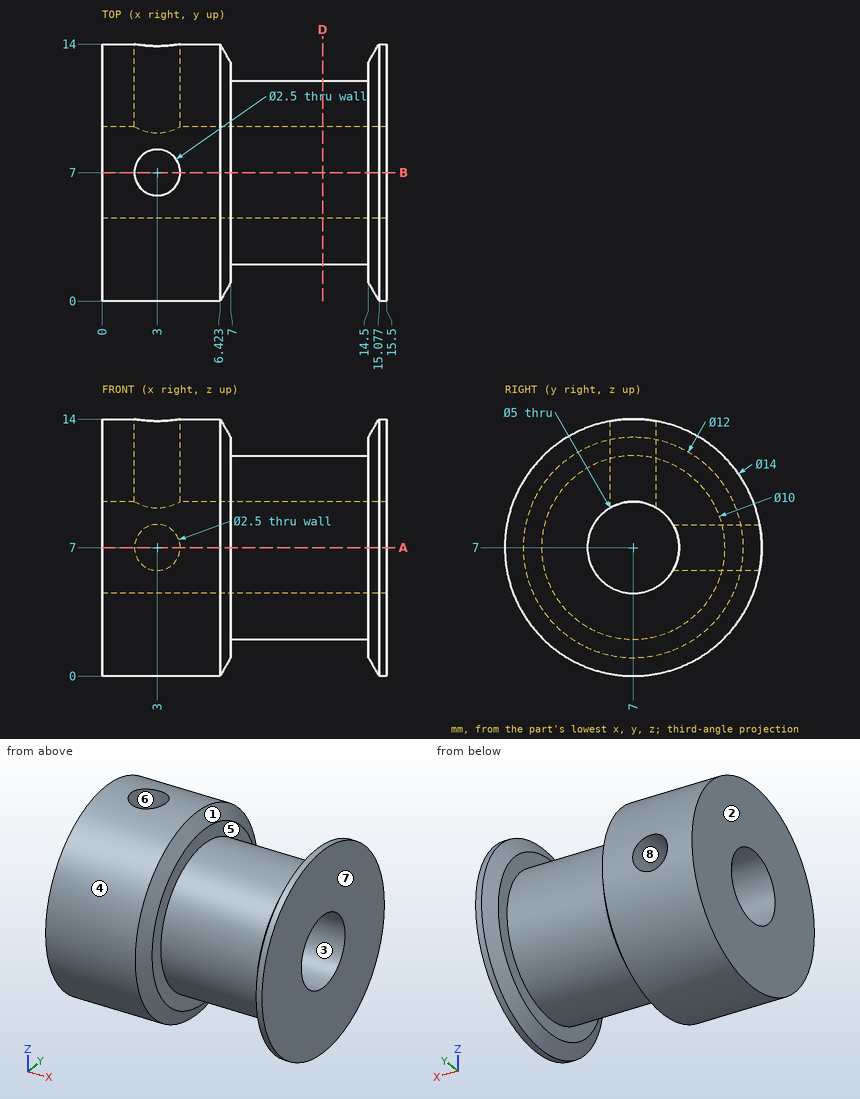
Verification items for this drawing (mm, ordinates from the low corner). A direction names the side the tool comes from. Give positions to 0.01 mm unless a question says otherwise; leave off trailing zeros. Loops run counter-clockwise (first coordinate to the right, second up) from the corner with the lowest first, then second, coordinate; pieces in that order, holes last. Notation, with made-up numbers: M 88.25,53 L 119.25,53 A16 cw 119.25,68 Z; hole C -25,73 d9. An arc over 180 degrees is marked long. Write item = value, one per line. Start each with the question number.
1. Draft check along Z on the marked faces 1, 2 and 3. Enter one of: +Z half, -Z half, draft (parallel to the pull), parting line (faces both ways), or undercut.
2. Section check A-A, the plane z = 7. Enter the section's corners in (x, y).
3. Go/stop test with flat-tipped pins: P1, Ø3, axis at x = 9.5, y = 8.5, coming from the +Z side; P2, Ø1.5, axis at x = 2.5, z = 12, coming from the -Y side. Record where each tip stops, or that it passes through.
4. Tool access check on the marked faces 4, 5, 6, 7 and 8. Record the directions out of +Z, -Z, +X, -X, +Y, -Y that give a thin tool (end or side, any length) a straight path to the whole face; none if there is none.
5. Thickness scan on probe 1 along X at (y, z) = (12.5, 7); probe 2 along X at (y, z) = (6.5, 13) (1 decimal); probe 3 along Y at (x, z) = (6.75, 6.25) (1 decimal). Record the ranges inside material, lowest first.
6. Section check D-D, the plane x = 12. Enter the section's corners in (y, z), plus the area to 3 significant figures.
Values follow:
q1.face_1 = parting line
q1.face_2 = draft
q1.face_3 = undercut
q2.outline = M 0,0 L 6.42,0 L 7,1 L 7,2 L 14.5,2 L 14.5,1 L 15.08,0 L 15.5,0 L 15.5,4.5 L 0,4.5 Z; M 0,9.5 L 1.75,9.5 L 1.75,14 L 0,14 Z; M 4.25,9.5 L 15.5,9.5 L 15.5,14 L 15.08,14 L 14.5,13 L 14.5,12 L 7,12 L 7,13 L 6.42,14 L 4.25,14 Z
q3.P1 = 12
q3.P2 = 1.44
q4.face_4 = +X, -X
q4.face_5 = none
q4.face_6 = +Z
q4.face_7 = +Z, -Z, +X, +Y, -Y
q4.face_8 = +Y
q5.probe_1 = 0 to 1.75, 4.25 to 7, 14.5 to 15.5
q5.probe_2 = 0 to 1.9, 4.1 to 7, 14.5 to 15.5
q5.probe_3 = 0.6 to 4.6, 9.4 to 13.4
q6.outline = C 7,7 d10; hole C 7,7 d5
q6.area = 58.9 mm^2
